Build history of the part. All positions in model axes, mm. A direction names the side the tool comes from. Coordinates: 2 decimals unless noted, no trailing zeros. Write each loop counter-clockwise with the first axis right and the second up, starting at its lowest first coordinate (ties: lowest second). Pieces come first, ordered by that corner, then holes.
```python
from build123d import *

# Parameters (mm, degrees)
BOSS_EXTRUDE1_DEPTH = 7.5
SKETCH2_R           = 2.5
BOSS_EXTRUDE2_DEPTH = 1
SKETCH3_R           = 0.5
BOSS_EXTRUDE3_DEPTH = 9
SKETCH4_W           = 12
SKETCH4_H           = 10
BOSS_EXTRUDE4_DEPTH = 1
SKETCH5_R           = 1.5
CUT_EXTRUDE1_DEPTH  = 26


with BuildPart() as part:
    # Sketch1 → Boss-Extrude1 (new body, symmetric)
    with BuildSketch(Plane.XY):
        with BuildLine():
            Line((-3.31662479, 5), (3.31662479, 5))
            ThreePointArc((3.31662479, 5), (6, 0), (3.31662479, -5))
            Line((3.31662479, -5), (-3.31662479, -5))
            ThreePointArc((-3.31662479, -5), (-6, 0), (-3.31662479, 5))
        make_face()
    extrude(amount=BOSS_EXTRUDE1_DEPTH, both=True)

    # Sketch2 → Boss-Extrude2 (add)
    with BuildSketch(Plane(origin=(0, 0, -7.5), x_dir=(-1, 0, 0), z_dir=(0, 0, -1))):
        Circle(SKETCH2_R)
    extrude(amount=BOSS_EXTRUDE2_DEPTH)

    # Sketch3 → Boss-Extrude3 (add)
    with BuildSketch(Plane.XY.offset(7.5)):
        with Locations((3.358757211, 3.358757211)):
            Circle(SKETCH3_R)
        with Locations((-3.358757211, -3.358757211)):
            Circle(SKETCH3_R)
    extrude(amount=BOSS_EXTRUDE3_DEPTH)

    # Sketch4 → Boss-Extrude4 (add)
    with BuildSketch(Plane.XY.offset(16.5)):
        Rectangle(SKETCH4_W, SKETCH4_H)
    extrude(amount=-BOSS_EXTRUDE4_DEPTH)

    # Sketch5 → Cut-Extrude1 (cut, through all)
    with BuildSketch(Plane.XY.offset(16.5)):
        Circle(SKETCH5_R)
    extrude(amount=-CUT_EXTRUDE1_DEPTH, mode=Mode.SUBTRACT)


solid = part.part
```
1. Saw through at A-A on x = 0. List the corners of the cut face in (y, z), plus the area to 3 significant figures.
Computed values:
outline: (-5, -7.5) - (-2.5, -7.5) - (-2.5, -8.5) - (-1.5, -8.5) - (-1.5, 7.5) - (-5, 7.5) - close; (-5, 15.5) - (-1.5, 15.5) - (-1.5, 16.5) - (-5, 16.5) - close; (1.5, -8.5) - (2.5, -8.5) - (2.5, -7.5) - (5, -7.5) - (5, 7.5) - (1.5, 7.5) - close; (1.5, 15.5) - (5, 15.5) - (5, 16.5) - (1.5, 16.5) - close
area: 114 mm2
2. 3-axis set-ups, long thin cutter, end or side, ignore diameter. For faces 1 (the face through (6, 0, 0)), 2 (the face through (0.54, -2.44, -7.99)), 3 (the face through (-3.467, -3.847, 11.444)): which of +Z, -Z, +X, -X, +Y, -Y reach the whole face in a straight line?
Computed values:
face 1: -Z, +X
face 2: -Z
face 3: none
3. Saw through at B-B on y = 0. List the corners of the cut face in (x, z), plus the area to 3 significant figures.
Computed values:
outline: (-6, -7.5) - (-2.5, -7.5) - (-2.5, -8.5) - (-1.5, -8.5) - (-1.5, 7.5) - (-6, 7.5) - close; (-6, 15.5) - (-1.5, 15.5) - (-1.5, 16.5) - (-6, 16.5) - close; (1.5, -8.5) - (2.5, -8.5) - (2.5, -7.5) - (6, -7.5) - (6, 7.5) - (1.5, 7.5) - close; (1.5, 15.5) - (6, 15.5) - (6, 16.5) - (1.5, 16.5) - close
area: 146 mm2
4. Flat gauge pins, fed straight in: pin 1 (1.5 mm diameter, centred on x = 3, z = 14, fed in from -Y); pin 2 (2.5 mm diameter, centred on x = 0, y = 0, fed in from +Z); pin 3 (2 mm diameter, centred on y = -4, z = 14, fed in from +X). Where does each tip first touch, or does it go through?
Computed values:
pin 1: stops at y = 2.86
pin 2: passes through
pin 3: stops at x = -2.86
5. Probe line 1 along Y through (x, z) = (0, 4); line 2 along Z through (x, y) = (-1.5, -3.25); line 3 along Z through (x, y) = (-0.75, 2.25). List the from-to ranges inside material, lowest first.
Computed values:
line 1: y = -5 to -1.5, 1.5 to 5
line 2: z = -7.5 to 7.5, 15.5 to 16.5
line 3: z = -8.5 to 7.5, 15.5 to 16.5
6. Mould opens along Y. For faces 4 (the face through (-1.5, 0.07, 16.01)), 5 (the face through (-6, 0, 16)), 6 (the face through (-6, 0, 0)) say: +Y half, -Y half, draft (parallel to the pull), parting line (faces both ways), or undercut.
Computed values:
face 4: undercut
face 5: draft
face 6: parting line
7. Saw through at C-C on x = -5. List the corners of the cut face in (y, z).
Computed values:
outline: (-5, 15.5) - (5, 15.5) - (5, 16.5) - (-5, 16.5) - close; (-3.32, -7.5) - (3.32, -7.5) - (3.32, 7.5) - (-3.32, 7.5) - close
8. Saw through at D-D on z = 9.25. List the corners of the cut face in (x, y), plus the area to 3 significant figures.
Computed values:
outline: circle Ø1 at (-3.36, -3.36); circle Ø1 at (3.36, 3.36)
area: 1.57 mm2
